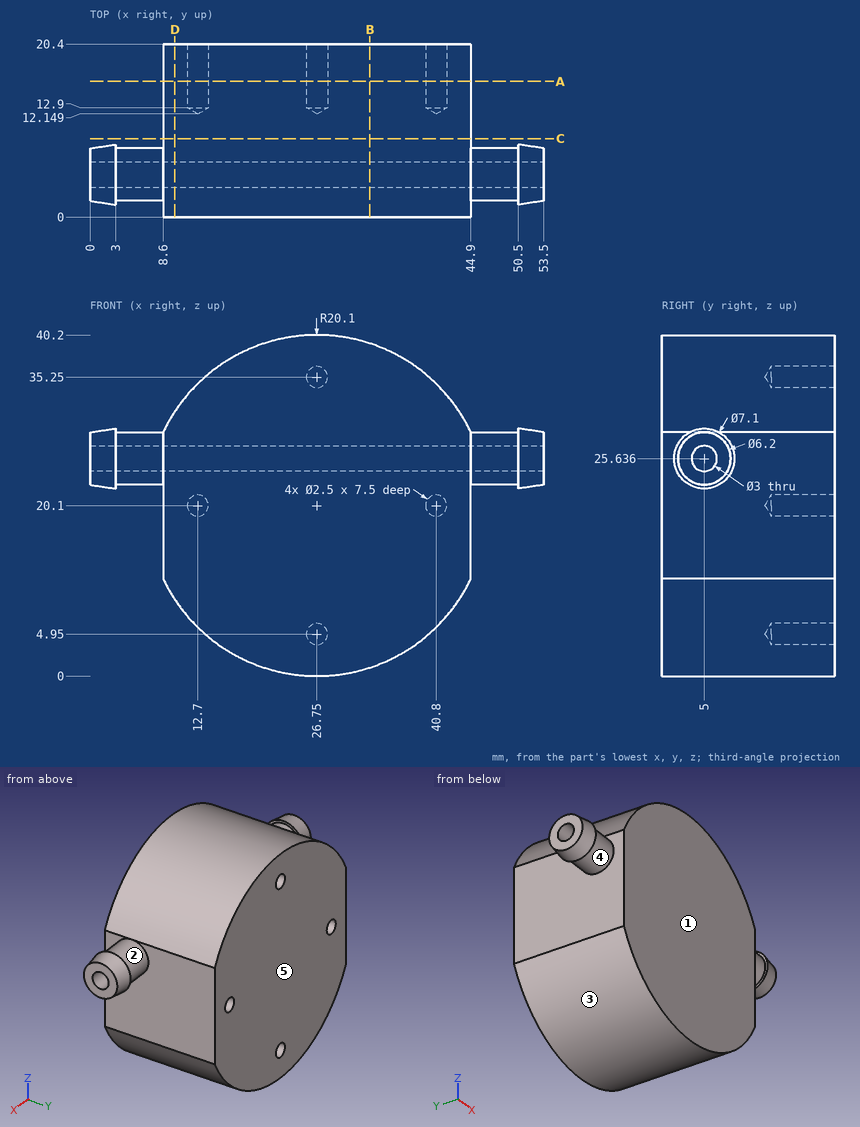
Could you check a few things on this drawing? It's one solid part, dimensions in mm from its lowest x, y, z. A direction names the side the tool comes from. Coordinates: 2 decimals unless noted, no trailing zeros. Order: outer loops, then holes, each group sorted by start corner. A loop starts at its lowest first (then second) coordinate and runs counter-clockwise, first axis right, second up.
1. If we section it at C-C (y = 9.25): Please give me the cut outline in (x, z).
2. If we section it at D-D (x = 10): Please give me the cut outline in (y, z), then the cut area to 3 significant figures.
3. I'm going to push flat-ended pins straight in: pin 1 (8.5 mm diameter, centred on y = 8, z = 23, fed in from -X); pin 2 (1.5 mm diameter, centred on y = 12, z = 11, fed in from -X); pin 3 (1.5 mm diameter, centred on y = 6.5, z = 10, fed in from -X); pin 4 (1 mm diameter, centred on x = 20.5, y = 17, fed in from +Z). Where does each tip first touch, or does it pass through?
4. Thinking about a two-plate mould opening in X: for the marked faces 1, 2 and 3, which applies, +X half, -X half, draft (parallel to the pull), parting line (faces both ways), or undercut?
5. If we section it at B-B (x = 33): Please give me the cut outline in (y, z), then the cut area to 3 significant figures.
6. For the marked faces 4 and 5, which set-ups out of +Z, -Z, +X, -X, +Y, -Y let a thin tool reach every point of the face, with its end or its side?
7. If we section it at A-A (y = 16): Please give me the cut outline in (x, z), then the cut area to 3 significant figures.
8. I need wall thicknesses on line 1 (X direction, y = 10, z = 13.5); line 2 (X direction, y = 18, z = 20.5) (1 decimal); line 3 (X direction, y = 17.5, z = 35.25). Which ranges of each line are inside material? Lowest first, please.
Entries:
1. outline: (8.6, 11.46) arc R20.1 ccw to (44.9, 11.46) - (44.9, 28.74) arc R20.1 ccw to (8.6, 28.74) - close
2. outline: (0, 8.99) - (20.4, 8.99) - (20.4, 31.21) - (0, 31.21) - close; hole circle Ø3 at (5, 25.64)
2. area: 446 mm2
3. pin 1: stops at x = 0
3. pin 2: stops at x = 8.6
3. pin 3: stops at x = 8.96
3. pin 4: stops at z = 39.36
4. face 1: draft
4. face 2: undercut
4. face 3: parting line
5. outline: (0, 1) - (20.4, 1) - (20.4, 39.2) - (0, 39.2) - close; hole circle Ø3 at (5, 25.64)
5. area: 772 mm2
6. face 4: none
6. face 5: +Z, -Z, +X, -X, +Y
7. outline: (8.6, 11.46) arc R20.1 ccw to (44.9, 11.46) - (44.9, 28.74) arc R20.1 ccw to (8.6, 28.74) - close; hole circle Ø2.5 at (12.7, 20.1); hole circle Ø2.5 at (26.75, 4.95); hole circle Ø2.5 at (26.75, 35.25); hole circle Ø2.5 at (40.8, 20.1)
7. area: 1,200 mm2
8. line 1: x = 8.6 to 44.9
8. line 2: x = 8.6 to 11.5, 13.9 to 39.6, 42 to 44.9
8. line 3: x = 13.54 to 25.5, 28 to 39.96
